The figure shows three views and two pictorial views of one solid part (mm, origin at its lowest corner). Answer the questions. A direction names the side the tool comes from. Coordinates: 2 decimals unless noted, no trailing zeros. Loops run counter-clockwise (first coordinate to the right, second up) from the corner with the lowest first, then second, coordinate; pieces in that order, holes last.
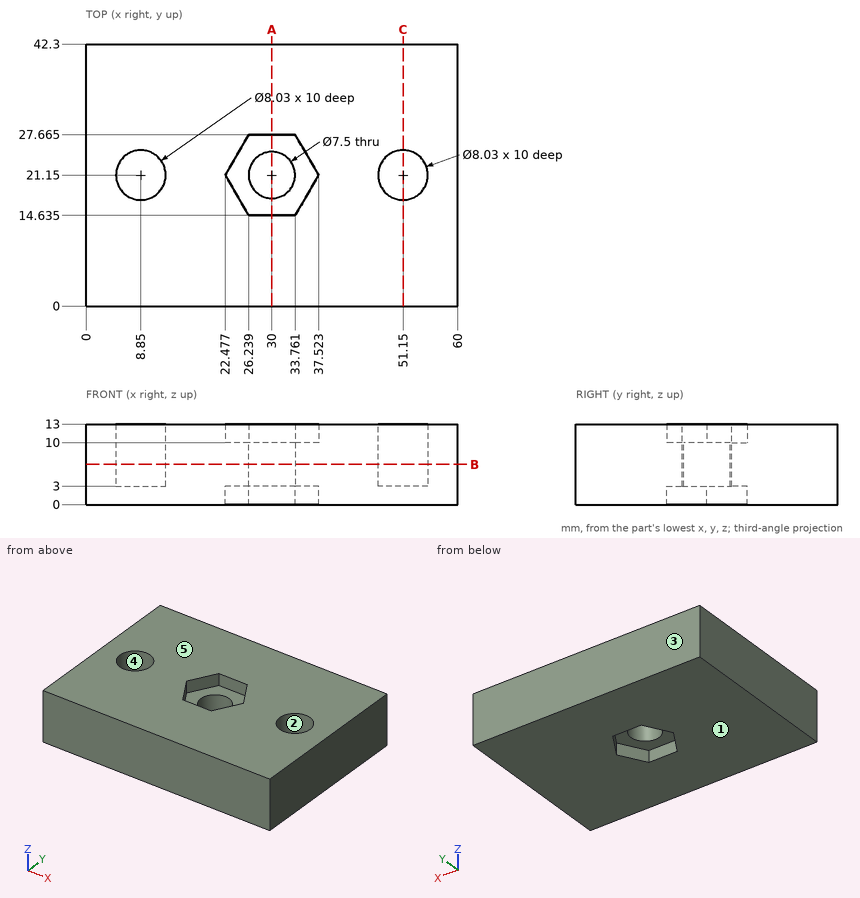
Q1. Straight lines are drawn through the part: probe 1 along Y at (x, z) = (51.15, 11) (1 decimal); probe 2 along X at (y, z) = (20.5, 6.75); probe 3 along Y at (x, z) = (30, 5.75). For each, find the intervals that lie inside material, in ascending order.
Findings below:
probe 1: y = 0 to 17.1, 25.2 to 42.3
probe 2: x = 0 to 4.89, 12.81 to 26.31, 33.69 to 47.19, 55.11 to 60
probe 3: y = 0 to 17.4, 24.9 to 42.3
Q2. Determine the mould class of the marked faces 3, 4 and 5 for opening direction Y: +Y half, -Y half, draft (parallel to the pull), parting line (faces both ways), or undercut.
Findings below:
face 3: +Y half
face 4: undercut
face 5: draft
Q3. A cutting plane is placed at C-C (x = 51.15). Give the vertices of the cut face in (y, z) (1 decimal).
Findings below:
outline: (0, 0) - (42.3, 0) - (42.3, 13) - (25.2, 13) - (25.2, 3) - (17.1, 3) - (17.1, 13) - (0, 13) - close
Q4. Which of the six approach directions +Z, -Z, +X, -X, +Y, -Y give full straight-line access (tool end or side, diameter ignored) to the marked faces 1 and 2?
Findings below:
face 1: -Z, +X, -X, +Y, -Y
face 2: +Z
Q5. A cutting plane is placed at A-A (x = 30). Give the vertices of the cut face in (y, z) (1 decimal).
Findings below:
outline: (0, 0) - (14.6, 0) - (14.6, 3) - (17.4, 3) - (17.4, 10) - (14.6, 10) - (14.6, 13) - (0, 13) - close; (24.9, 3) - (27.7, 3) - (27.7, 0) - (42.3, 0) - (42.3, 13) - (27.7, 13) - (27.7, 10) - (24.9, 10) - close
Q6. A cutting plane is placed at B-B (z = 6.5). Count the separate pieces of the cut face and the enclosed holes in it, then the cut area to 3 significant figures.
Findings below:
separate pieces: 1
enclosed holes: 3
area: 2,390 mm2
Q7. Flat-ended cylindrical pins translate along their axes: pin 1 Ø12 at (x, y) = (30, 21.15) entering from +Z; pin 2 Ø6.5 at (x, y) = (51.15, 21.15) entering from +Z; pin 3 Ø4 at (x, y) = (33, 21.5) entering from -Z. Find the tip coordinate at first contact, or state that the pin passes through.
Findings below:
pin 1: stops at z = 10
pin 2: stops at z = 3
pin 3: stops at z = 3
